For this review, take the finished solid that the model builds, in its own axes (mm). A direction names the side the tool comes from. Coordinates: 2 decimals unless noted, no trailing zeros. Loops run counter-clockwise (first coordinate to the right, second up) from the corner with the lowest first, then second, coordinate; pieces in that order, holes last. Notation, with made-up numbers: M 84.25,-26.75 L 101.25,-26.75 A8 cw 101.25,-17.75 Z; hole C -20.75,26 d2. An arc over 180 degrees is marked long. Write item = value, one per line.
Solid Edge part; units mm, degrees
sketch "Sketch1" plane through (0, 0, 0) normal (0, -1, 0) x (1, 0, 0)
  circle A0 centre (0, 0) radius 8
extrude "Protrusion1" add sketch "Sketch1" along normal mid plane 20.5
sketch "Sketch2" plane through (0, 0, 0) normal (0, -1, 0) x (1, 0, 0)
  line L0 (0, 10.9697) -> (-9.5, 5.4848)
  line L1 (-9.5, 5.4848) -> (-9.5, -5.4848)
  line L2 (-9.5, -5.4848) -> (0, -10.9697)
  line L3 (0, -10.9697) -> (9.5, -5.4848)
  line L4 (9.5, -5.4848) -> (9.5, 5.4848)
  line L5 (9.5, 5.4848) -> (0, 10.9697)
extrude "ExtrudedProtrusion_2" add sketch "Sketch2" along normal blind 2
Q1. Add section B-B (x = -6). Write out the cut boundary in (y, z), and give its area (3 significant figures).
Solved:
outline = M -10.25,-5.29 L -2,-5.29 L -2,-7.51 L 0,-7.51 L 0,-5.29 L 10.25,-5.29 L 10.25,5.29 L 0,5.29 L 0,7.51 L -2,7.51 L -2,5.29 L -10.25,5.29 Z
area = 226 mm²
Q2. Add section D-D (z = -8.75). Write out the cut boundary in (x, y).
Solved:
outline = M -3.84,-2 L 3.84,-2 L 3.84,0 L -3.84,0 Z
Q3. For line 1 along X through (y, z) = (5, 0.25); line 2 along Y through (x, z) = (-7.5, -4.5), list the stretches that pass through material, from the lowest coordinate up.
Solved:
line_1 = -8 to 8
line_2 = -2 to 0
Q4. For pin 1 Ø5 at (y, z) = (-5.5, -6.5) entering from +X; pin 2 Ø2 at (x, y) = (-3, 2.5) entering from -Z; pin 3 Ø3 at (x, y) = (-3, 5) entering from +Z, all flat-tipped, find the tip position at first contact; note any pin that passes through.
Solved:
pin_1 = 6.93
pin_2 = -7.75
pin_3 = 7.86
Q5. Add section A-A (z = 0). Write out the cut boundary in (x, y), and give its area (3 significant figures).
Solved:
outline = M -9.5,-2 L -8,-2 L -8,-10.25 L 8,-10.25 L 8,-2 L 9.5,-2 L 9.5,0 L 8,0 L 8,10.25 L -8,10.25 L -8,0 L -9.5,0 Z
area = 334 mm²
Q6. Add section C-C (y = 3.5). Write out the cut boundary in (x, z).
Solved:
outline = C 0,0 d16
Q7. Machinability: for faces 1 (the face through (-8, -2, -2)), 2 (the face through (-1.73, 5.05, -7.81)), 3 (the face through (0, -10.25, 0)), which of the approach directions +Z, -Z, +X, -X, +Y, -Y give a long, thin tool a straight path to every point of the face, cutting with its end or side? Answer none if there is none.
Solved:
face_1 = -Y
face_2 = +Y
face_3 = +Z, -Z, +X, -X, -Y
